Geometry check sheet. Reference: drawing and pictorial views, mm from the part's lowest x, y, z. Give positions to 0.01 mm unless a question says otherwise; leave off trailing zeros. Write each loop counter-clockwise with the first axis right and the second up, starting at its lowest first coordinate (ties: lowest second). Pieces come first, ordered by that corner, then holes. Notation, with made-up numbers: M 68.25,41.25 L 115.25,41.25 A15 cw 115.25,69.25 Z; hole C -22.5,15 d9. An arc over 180 degrees is marked long. Write each question's results on one line, items separated by ' | '. Start each with the question number.
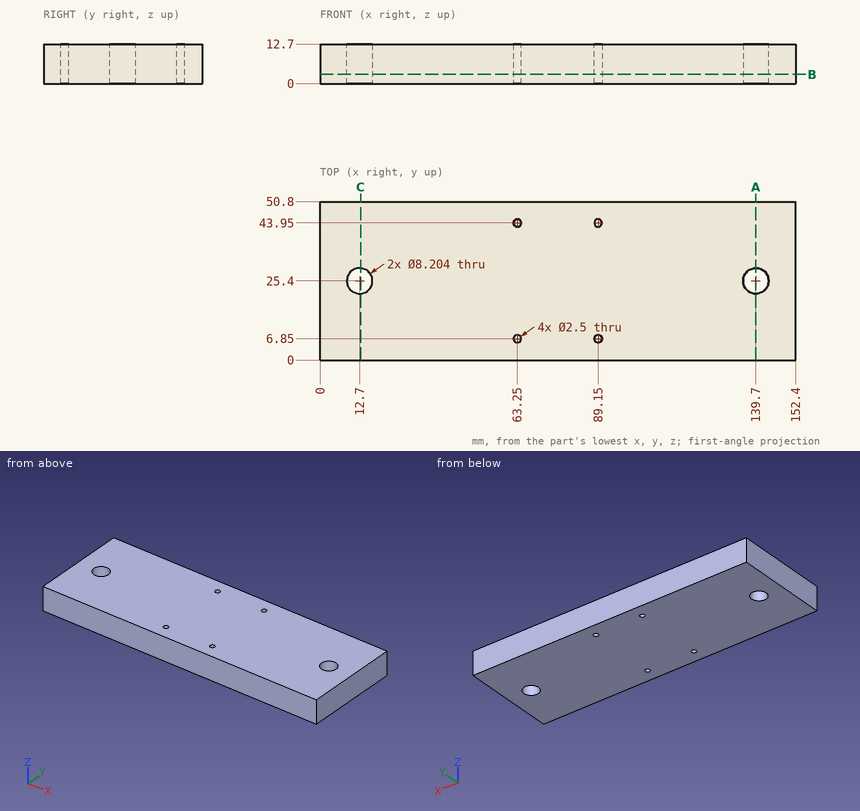
Q1. Section check C-C on x = 13. Record the boundary of the cut face in (y, z).
Q2. Section check A-A on x = 139.7. Record the boundary of the cut face in (y, z), plus the area to 3 significant figures.
Q3. Depth check by flat-ended pin: pin 1 Ø7.5 at (x, y) = (139.7, 25.4) entering from +Z. Enter the tip coordinate at first touch or a pass-through.
Q4. Section check B-B on z = 3. Record the boundary of the cut face in (x, y).
Q5. Scan lines: L1, parallel to Y at x = 89.15, z = 6.75; L2, parallel to X at y = 43.95, z = 4; L3, parallel to X at y = 43.5, z = 7.25. Record each from-to range of solid material in increasing order.
Check result:
1) outline: M 0,0 L 21.31,0 L 21.31,12.7 L 0,12.7 Z; M 29.49,0 L 50.8,0 L 50.8,12.7 L 29.49,12.7 Z
2) outline: M 0,0 L 21.3,0 L 21.3,12.7 L 0,12.7 Z; M 29.5,0 L 50.8,0 L 50.8,12.7 L 29.5,12.7 Z | area: 541 mm^2
3) pin 1: through
4) outline: M 0,0 L 152.4,0 L 152.4,50.8 L 0,50.8 Z; hole C 12.7,25.4 d8.2; hole C 63.25,6.85 d2.5; hole C 63.25,43.95 d2.5; hole C 89.15,6.85 d2.5; hole C 89.15,43.95 d2.5; hole C 139.7,25.4 d8.2
5) L1: 0 to 5.6, 8.1 to 42.7, 45.2 to 50.8 | L2: 0 to 62, 64.5 to 87.9, 90.4 to 152.4 | L3: 0 to 62.08, 64.42 to 87.98, 90.32 to 152.4
